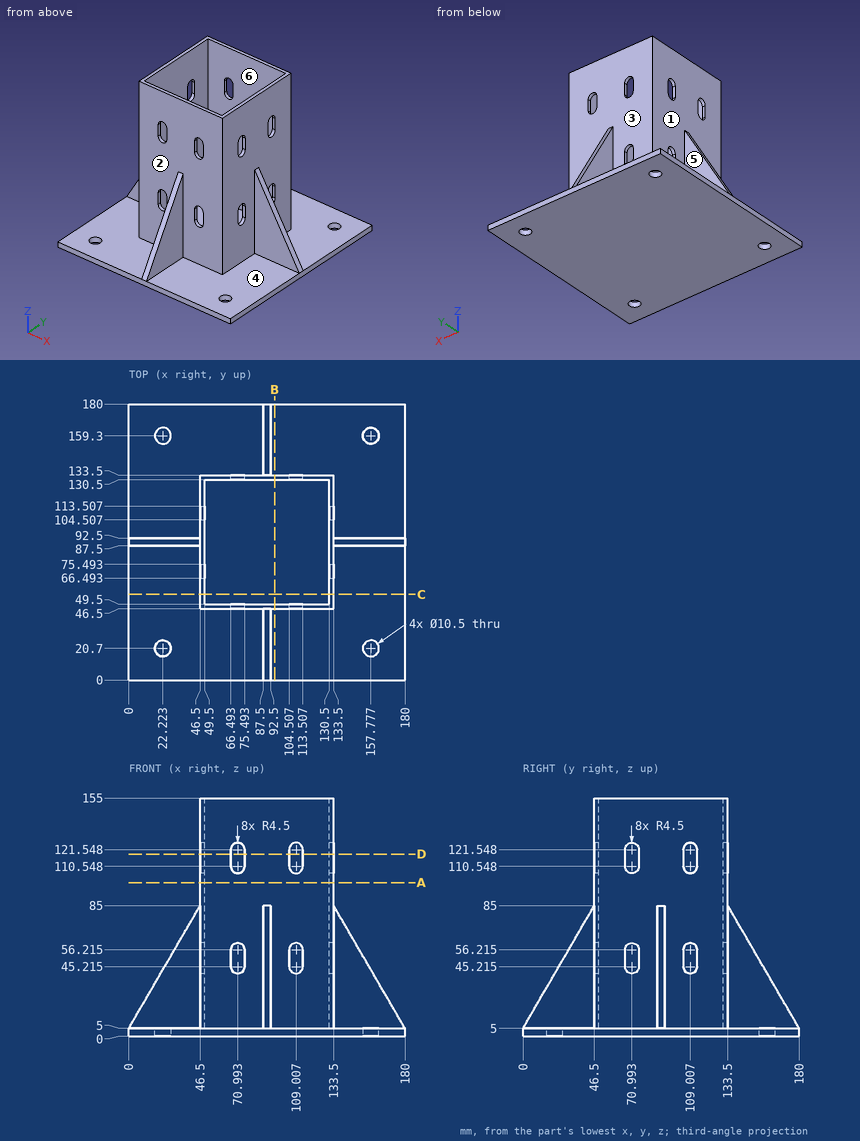
Geometry: see drawing. Coordinates: mm, zero at the bounding-box minimum. A direction names the side the tool comes from. Coordinates: 2 decimals unless noted, no trailing zeros. Loops run counter-clockwise (first coordinate to the right, second up) from the corner with the lowest first, then second, coordinate; pieces in that order, holes last. Notation, with made-up numbers: (-14, 2) - (-9, 2) arc R13 cw to (-9, 9) - close; hole circle Ø3 at (-37.5, 8). An arc over 180 degrees is marked (long way). Answer in a Markdown table with one row per item.
(1) Cut plane B-B on x = 95. Output: boundary loops of the cut face in (y, z), plus the area to 3 significant figures.
Model answer:
| item | result |
|---|---|
| outline | (0, 0) - (180, 0) - (180, 5) - (133.5, 5) - (133.5, 155) - (130.5, 155) - (130.5, 5) - (49.5, 5) - (49.5, 155) - (46.5, 155) - (46.5, 5) - (0, 5) - close |
| area | 1,800 mm² |
(2) Mould query, pull axis Y, two halves, no side actions, for the marked faces 4, 5 and 6. Classes: pulls with the +Y half, pulls with the -Y half, needs draft (parallel to the pull), parting line crosses it, or undercut.
Model answer:
| item | result |
|---|---|
| face 4 | needs draft |
| face 5 | pulls with the +Y half |
| face 6 | undercut |
(3) Cut plane A-A on z = 100. Output: boundary loops of the cut face in (x, y), plus the area to 3 significant figures.
Model answer:
| item | result |
|---|---|
| outline | (46.5, 46.5) - (133.5, 46.5) - (133.5, 133.5) - (46.5, 133.5) - close; hole (49.5, 49.5) - (130.5, 49.5) - (130.5, 130.5) - (49.5, 130.5) - close |
| area | 1,010 mm² |
(4) Cut plane D-D on z = 118.5. Count the separate pieces of the cut face and the enclosed holes in it.
Model answer:
| item | result |
|---|---|
| separate pieces | 8 |
| enclosed holes | 0 |
(5) Set-up query: the marked faces 1, 2 and 3. Return all of +Z, -Z, +X, -X, +Y, -Y with unobstructed straight access to the full face (end or side cutting, diameter ignored); none if empty.
Model answer:
| item | result |
|---|---|
| face 1 | +Z, -X |
| face 2 | +Z, -Y |
| face 3 | +Z, +Y |
(6) Pin query (flat end, axial travel): P1, Ø24.5, axis at y = 72.5, z = 93.5, coming from the -X side; P2, Ø2, axis at x = 94.5, z = 121.5, coming from the -Y side; P3, Ø3.5, axis at x = 48, z = 117, coming from the +Y side; P4, Ø23.5, axis at x = 20.5, z = 65, coming from the +Y side. Return the tip coordinate at first contact, or that it passes through.
Model answer:
| item | result |
|---|---|
| P1 | stops at x = 46.5 |
| P2 | stops at y = 46.5 |
| P3 | stops at y = 133.5 |
| P4 | passes through |
(7) Material intervals for L1, parallel to X at y = 94, z = 11; L2, parallel to Z at x = 137.5, y = 95.5, sorted ascending. Write a range as from..to.
Model answer:
| item | result |
|---|---|
| L1 | x = 46.5..49.5, 130.5..133.5 |
| L2 | z = 0..5 |
